```python
from build123d import *

# Parameters (mm, degrees)
IZIM1_R                     = 13.95
IZIM1_R_2                   = 4
Y_KSEKLIK_EKSTR_ZYON3_DEPTH = 6
M3_BO_LUKLU_DELIK3_D        = 3.2
KES_EKSTR_ZYON2_DEPTH       = 6
DAIRESEL_KAPLAMA1_COUNT     = 2
DAIRESEL_KAPLAMA1_ANGLE     = 90
KES_EKSTR_ZYON11_DEPTH      = 4.7
PAH1_SIZE                   = 2
KES_EKSTR_ZYON12_START      = -4.7
KES_EKSTR_ZYON12_DEPTH      = 4.7
DAIRESEL_KAPLAMA2_COUNT     = 3
DAIRESEL_KAPLAMA2_ANGLE     = 180


with BuildPart() as part:
    # Çizim1 → Yükseklik-Ekstrüzyon3 (new body)
    with BuildSketch(Plane.XY):
        Circle(IZIM1_R)
        Circle(IZIM1_R_2, mode=Mode.SUBTRACT)
    extrude(amount=Y_KSEKLIK_EKSTR_ZYON3_DEPTH)

    # M3 Boşluklu Delik3 (through all)
    with Locations(Plane(origin=(0, 0, 0), x_dir=(-1, 0, 0), z_dir=(0, 0, -1))):
        with Locations((-5.656854249, 5.656854249), (-6.717514421, -6.717514421), (5.656854249, -5.656854249), (6.717514421, 6.717514421)):
            Hole(M3_BO_LUKLU_DELIK3_D / 2)

    # Çizim13 → Kes-Ekstrüzyon2 (cut)
    with BuildSketch(Plane.XY.offset(6)):
        with BuildLine():
            ThreePointArc((-10.129468154, 3.782692346), (-10.95644466, -0.028335886), (-9.925054528, -3.789194927))
            ThreePointArc((-9.925054528, -3.789194927), (-8.496760909, -4.195368951), (-8.090586885, -2.767075332))
            ThreePointArc((-8.090586885, -2.767075332), (-8.857209488, 0.028335886), (-8.242525614, 2.861037394))
            ThreePointArc((-8.242525614, 2.861037394), (-8.725169408, 4.26533614), (-10.129468154, 3.782692346))
        make_face()
        with BuildLine():
            ThreePointArc((10.129468154, 3.782692346), (10.95644466, -0.028335886), (9.925054528, -3.789194927))
            ThreePointArc((9.925054528, -3.789194927), (8.496760909, -4.195368951), (8.090586885, -2.767075332))
            ThreePointArc((8.090586885, -2.767075332), (8.857209488, 0.028335886), (8.242525614, 2.861037394))
            ThreePointArc((8.242525614, 2.861037394), (8.725169408, 4.26533614), (10.129468154, 3.782692346))
        make_face()
    kes_ekstr_zyon2 = extrude(amount=-KES_EKSTR_ZYON2_DEPTH, mode=Mode.SUBTRACT)

    # Dairesel Kaplama1: Kes-Ekstrüzyon2 ×2 about axis
    dairesel_kaplama1_axis = Axis((0, 0, 0), (0, 0, 1))
    for i in range(1, DAIRESEL_KAPLAMA1_COUNT):
        add(kes_ekstr_zyon2.rotate(dairesel_kaplama1_axis, i * DAIRESEL_KAPLAMA1_ANGLE / (DAIRESEL_KAPLAMA1_COUNT - 1)), mode=Mode.SUBTRACT)

    # Çizim16 → Kes-Ekstrüzyon11 (cut)
    with BuildSketch(Plane.XY.offset(6)):
        with BuildLine():
            Line((-6.125352388, 12.533258081), (-4.26533614, 8.725169408))
            ThreePointArc((-4.26533614, 8.725169408), (-4.314854036, 9.527277584), (-3.782692346, 10.129468154))
            ThreePointArc((-3.782692346, 10.129468154), (0.028335886, 10.95644466), (3.789194927, 9.925054528))
            ThreePointArc((3.789194927, 9.925054528), (4.288091233, 9.295029113), (4.195368951, 8.496760909))
            Line((4.195368951, 8.496760909), (6.374759269, 12.408261129))
            ThreePointArc((6.374759269, 12.408261129), (0.139488378, 13.949302599), (-6.125352388, 12.533258081))
        make_face()
    extrude(amount=-KES_EKSTR_ZYON11_DEPTH, mode=Mode.SUBTRACT)

    # Pah1
    pah1_edges = [part.edges().sort_by_distance(p)[0] for p in [
        (-7.387619176, -11.833240592, 6),
    ]]
    chamfer(pah1_edges, length=PAH1_SIZE)

    # Çizim18 → Kes-Ekstrüzyon12 (cut)
    with BuildSketch(Plane.XY.offset(6).offset(KES_EKSTR_ZYON12_START)):
        with BuildLine():
            Line((-10.735839815, 5.248260994), (-12.53263309, 6.126631034))
            ThreePointArc((-12.53263309, 6.126631034), (-13.94997085, -0.028518286), (-12.50747878, -6.177821183))
            Line((-12.50747878, -6.177821183), (-10.714291858, -5.292112053))
            ThreePointArc((-10.714291858, -5.292112053), (-11.949975029, -0.024429643), (-10.735839815, 5.248260994))
        make_face()
    kes_ekstr_zyon12 = extrude(amount=KES_EKSTR_ZYON12_DEPTH, mode=Mode.SUBTRACT)

    # Dairesel Kaplama2: Kes-Ekstrüzyon12 ×3 about axis
    dairesel_kaplama2_axis = Axis((0, 0, 6), (0, 0, 1))
    for i in range(1, DAIRESEL_KAPLAMA2_COUNT):
        add(kes_ekstr_zyon12.rotate(dairesel_kaplama2_axis, i * DAIRESEL_KAPLAMA2_ANGLE / (DAIRESEL_KAPLAMA2_COUNT - 1)), mode=Mode.SUBTRACT)


solid = part.part
```
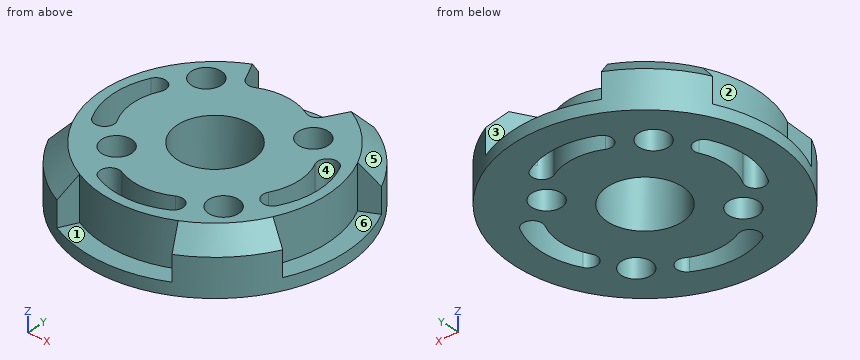
Can you work these out from the model? Positions are in its coordinate system, mm. Face numbers are marked on the shaded views. A direction names the side the tool comes from. Give positions to 0.01 mm unless a question says otherwise; leave off trailing zeros. Loops run counter-clockwise (first coordinate to the right, second up) from the corner with the lowest first, then second, coordinate; pieces in that order, holes last. Notation, with made-up numbers: M 0,76 L 6,76 A19 cw 6,81 Z; hole C 38,40.5 d9. An arc over 180 degrees is marked long. Use one line per item in the form item = value. Start each with the question number.
(1) Please list where these lines run through material, in increasing order: line 1 (Y direction, x = 0, z = 3.95); line 2 (X direction, y = 3.25, z = 3.75); line 3 (Y direction, x = 1.25, z = 1.15).
(2) I'm going to push flat-ended pins straight in: P1, Ø3, axis at x = 9.5, z = 1.5, coming from the -Y side; P2, Ø1.5, axis at y = 1.5, z = 3, coming from the +X side; P3, Ø1.5, axis at x = -0.5, y = 10, coming from the +Z side; P4, Ø3, axis at y = 5.5, z = 3, coming from the -X side. Where does each tip first touch, or does it pass through?
(3) I want a section at B-B, the plane y = 0. Write out the boundary of the cut face in (x, z).
(4) I want a section at A-A, the plane z = 0.4. State how many separate pieces and enclosed holes the cut face has, and give its area (3 significant figures).
(5) On a 3-axis mill with a long thin cutter (end or side, diameter ignored), from which of +Z, -Z, +X, -X, +Y, -Y can I reach the whole of each face in a straight line? I mean the marked faces 1, 2 and 3. Say none if no direction works.
(6) I want a section at C-C, the plane x = 0. Write out the boundary of the cut face in (y, z).
(7) Thinking about a two-plate mould opening in X: for the marked faces 4, 5 and 6, which applies, released by +X, released by -X, zero draft, split by the parting line, or undercut?
Worked out:
q1.line_1 = -11.95 to -10.96, -8.86 to -4, 4 to 8.86
q1.line_2 = -11.5 to -10.37, -8.14 to -2.33, 2.33 to 8.14, 10.37 to 11.5
q1.line_3 = -13.89 to -10.83, -8.69 to -3.8, 3.8 to 8.69, 10.83 to 13.89
q2.P1 = -11.43
q2.P2 = 11.93
q2.P3 = through
q2.P4 = -12.53
q3.outline = M -13.95,0 L -10.96,0 L -10.96,6 L -11.95,6 L -11.95,1.3 L -13.95,1.3 Z; M -8.86,0 L -4,0 L -4,6 L -8.86,6 Z; M 4,0 L 8.86,0 L 8.86,6 L 4,6 Z; M 10.96,0 L 13.95,0 L 13.95,1.3 L 11.95,1.3 L 11.95,6 L 10.96,6 Z
q4.separate_pieces = 1
q4.enclosed_holes = 9
q4.area = 457 mm²
q5.face_1 = +Z, -Y
q5.face_2 = +Z, -X
q5.face_3 = +Z, +Y
q6.outline = M -13.95,0 L -10.96,0 L -10.96,6 L -11.95,6 L -11.95,1.3 L -13.95,1.3 Z; M -8.86,0 L -4,0 L -4,6 L -8.86,6 Z; M 4,0 L 8.86,0 L 8.86,6 L 4,6 Z; M 10.96,0 L 13.95,0 L 13.95,1.3 L 10.96,1.3 Z
q7.face_4 = undercut
q7.face_5 = released by +X
q7.face_6 = zero draft
